The listing builds one solid part. Answer for the finished solid, in the listing's coordinates (mm). A direction names the side the tool comes from. Coordinates: 2 decimals unless noted, no trailing zeros. Loops run counter-clockwise (first coordinate to the right, second up) from the corner with the lowest first, then second, coordinate; pieces in that order, holes last. Notation, with made-up numbers: (13, 55.25) -> (36, 55.25) arc R28 ccw to (36, 93.25) -> close; hole circle Ø5 at (49, -6). An arc over 180 degrees is marked (long way). Answer in a Markdown table with one row per item.
```python
from build123d import *

# Parameters (mm, degrees)
SKETCH052_W            = 600
SKETCH052_H            = 60
PAD003_DEPTH           = 400
SKETCH004_W            = 612
SKETCH004_H            = 50
PAD004_DEPTH           = 406
SKETCH053_W            = 712
SKETCH053_H            = 912
PAD005_DEPTH           = 6
CUT001_PLACEMENT_ANGLE = 180


with BuildPart() as body002:
    # Sketch052 → Pad003 (new body, symmetric)
    with BuildSketch(Plane.XZ):
        with Locations((0, 30)):
            Rectangle(SKETCH052_W, SKETCH052_H)
    extrude(amount=PAD003_DEPTH, both=True)


with BuildPart() as cut001:
    # Sketch004 → Pad004 (new body, symmetric)
    with BuildSketch(Plane.XZ):
        with Locations((0, 25)):
            Rectangle(SKETCH004_W, SKETCH004_H)
    extrude(amount=PAD004_DEPTH, both=True)

    # Sketch053 (on Face3 of Pad004) → Pad005 (join)
    with BuildSketch(Plane(origin=(0, 0, 50), x_dir=(-1, 0, 0), z_dir=(0, 0, 1))):
        Rectangle(SKETCH053_W, SKETCH053_H)
    extrude(amount=PAD005_DEPTH)

    # Cut001: cut Body002
    add(body002.part, mode=Mode.SUBTRACT)


with BuildPart() as cut001_1:
    # Cut001 placement: moved
    add(cut001.part.rotate(Axis((0, 0, 0), (0, 1, 0)), CUT001_PLACEMENT_ANGLE))


solid = cut001_1.part
```
Item 1: A cutting plane is placed at B-B, the plane x = 23. Determine the outline of the cut face in (y, z), plus the area to 3 significant figures.
Findings below:
| item | result |
|---|---|
| outline | (-456, -56) -> (-400, -56) -> (-400, 0) -> (-406, 0) -> (-406, -50) -> (-456, -50) -> close; (400, -56) -> (456, -56) -> (456, -50) -> (406, -50) -> (406, 0) -> (400, 0) -> close |
| area | 1,270 mm2 |
Item 2: A cutting plane is placed at A-A, the plane y = 380. Determine the outline of the cut face in (x, z), plus the area to 3 significant figures.
Findings below:
| item | result |
|---|---|
| outline | (-356, -56) -> (-300, -56) -> (-300, 0) -> (-306, 0) -> (-306, -50) -> (-356, -50) -> close; (300, -56) -> (356, -56) -> (356, -50) -> (306, -50) -> (306, 0) -> (300, 0) -> close |
| area | 1,270 mm2 |
Item 3: Flat-ended cylindrical pins translate along their axes: pin 1 Ø1.5 at (y, z) = (139.5, -8.5) entering from +X; pin 2 Ø25 at (x, z) = (-113, -27.5) entering from +Y; pin 3 Ø15 at (x, z) = (7.5, -27.5) entering from -Y. Find the tip coordinate at first contact, or state that the pin passes through.
Findings below:
| item | result |
|---|---|
| pin 1 | stops at x = 306 |
| pin 2 | stops at y = 406 |
| pin 3 | stops at y = -406 |
Item 4: Find the intervals of material crossed by probe 1 along X at (y, z) = (155.5, -23.5); probe 2 along Y at (x, z) = (213.5, -20.5); probe 3 along Y at (x, z) = (-255, -51), in increasing order.
Findings below:
| item | result |
|---|---|
| probe 1 | x = -306 to -300, 300 to 306 |
| probe 2 | y = -406 to -400, 400 to 406 |
| probe 3 | y = -456 to -400, 400 to 456 |
Item 5: Determine the mould class of faces 1 (the face through (306, -6, -25)), 2 (the face through (-318, -2, -56)), 3 (the face through (300, -6, -28)) for opening direction X: +X half, -X half, draft (parallel to the pull), parting line (faces both ways), or undercut.
Findings below:
| item | result |
|---|---|
| face 1 | +X half |
| face 2 | draft |
| face 3 | undercut |
Item 6: A cutting plane is placed at C-C, the plane z = -36.5. Determine the outline of the cut face in (x, y), plus the area to 3 significant figures.
Findings below:
| item | result |
|---|---|
| outline | (-306, -406) -> (306, -406) -> (306, 406) -> (-306, 406) -> close; hole (-300, -400) -> (300, -400) -> (300, 400) -> (-300, 400) -> close |
| area | 16,900 mm2 |
Item 7: A tool of negligible diameter and unlimited length cuts with its end or side. For faces 4 (the face through (-300, -6, -28)), 5 (the face through (4, -406, -25)), 6 (the face through (4, 406, -25)), 7 (the face through (-306, -6, -25)), from which of +Z, -Z, +X, -X, +Y, -Y can it reach the whole face along a straight path? Write none if from no direction.
Findings below:
| item | result |
|---|---|
| face 4 | +Z, -Z |
| face 5 | +Z, +X, -X, -Y |
| face 6 | +Z, +X, -X, +Y |
| face 7 | +Z, -X, +Y, -Y |
